```python
from build123d import *

# Parameters (mm, degrees)
F0_R     = 37
F0_R_2   = 3.25
F1_DEPTH = 4
F2_SIZE  = 2.75
F3_SIZE  = 0.5


with BuildPart() as f1:
    # F0 (on Top) → F1 (new body)
    with BuildSketch(Plane.XY):
        Circle(F0_R)
        with Locations((0, -29)):
            Circle(F0_R_2, mode=Mode.SUBTRACT)
        with Locations((-29, 0)):
            Circle(F0_R_2, mode=Mode.SUBTRACT)
        with Locations((29, 0)):
            Circle(F0_R_2, mode=Mode.SUBTRACT)
        with Locations((0, 29)):
            Circle(F0_R_2, mode=Mode.SUBTRACT)
    extrude(amount=F1_DEPTH)

    # F2
    f2_edges = [f1.edges().sort_by_distance(p)[0] for p in [
        (-3.25, -29, 4),
        (-32.25, 0, 4),
        (-3.25, 29, 4),
        (25.75, 0, 4),
    ]]
    chamfer(f2_edges, length=F2_SIZE)

    # F3
    f3_edges = [f1.edges().sort_by_distance(p)[0] for p in [
        (37, 0, 2),
        (-37, 0, 0),
        (-37, 0, 4),
        (-3.25, -29, 0),
        (-32.25, 0, 0),
        (-3.25, 29, 0),
        (25.75, 0, 0),
    ]]
    chamfer(f3_edges, length=F3_SIZE)


solid = f1.part
```
Verification items for the finished model (mm, model axes). Round coordinates to 2 decimals unless told otherwise and drop trailing zeros. Write each loop counter-clockwise with the first axis right and the second up, starting at its lowest first coordinate (ties: lowest second). Pieces come first, ordered by that corner, then holes. Notation, with made-up numbers: (-29.5, 34) - (-5.5, 34) arc R22 ccw to (-5.5, 48) - close; hole circle Ø9 at (20, 21.25). An arc over 180 degrees is marked (long way). Answer as a JSON object with one key per item and string values. Group by question number.
Q1. Section check C-C, the plane z = 2.45. Enter the section's corners in (x, y), plus the area to 3 significant figures.
Q2. Mould release check, pull along X, two halves, no side actions. Record for faces 1 (the cylindrical face through (-8.02, -36.12, 1.98)), 2 (the conical face through (32.26, 1.03, 1.42)), 3 (the flat face through (-1, 1, 0)): released by +X, released by -X, zero draft, split by the parting line, or undercut.
Q3. Section check A-A, the plane y = 0. Enter the section's corners in (x, z), plus the area to 3 significant figures.
Q4. Thickness scan on line 1 (Y direction, x = 0, z = 0.85); line 2 (X direction, y = 1, z = 1.7); line 3 (Y direction, x = 1.5, z = 3.6). Record the ranges inside material, lowest first.
Q5. Go/stop test with flat-tipped pins: pin 1 Ø1 at (x, y) = (-0.5, -5) entering from -Z; pin 2 Ø8.5 at (x, y) = (0, 29) entering from +Z; pin 3 Ø10.5 at (x, y) = (0, -29) entering from +Z; pin 4 Ø7.5 at (x, y) = (-29, 0) entering from +Z. Record where each tip stops, or that it passes through.
Found:
{
 "1": {"outline": "circle Ø74 at (0, 0); hole circle Ø8.9 at (-29, 0); hole circle Ø8.9 at (0, -29); hole circle Ø8.9 at (0, 29); hole circle Ø8.9 at (29, 0)", "area": "4,050 mm^2"},
 "2": {"face 1": "split by the parting line", "face 2": "undercut", "face 3": "zero draft"},
 "3": {"outline": "(-37, 0.5) - (-36.5, 0) - (-32.75, 0) - (-32.25, 0.5) - (-32.25, 1.25) - (-35, 4) - (-36.5, 4) - (-37, 3.5) - close; (-25.75, 0.5) - (-25.25, 0) - (25.25, 0) - (25.75, 0.5) - (25.75, 1.25) - (23, 4) - (-23, 4) - (-25.75, 1.25) - close; (32.25, 0.5) - (32.75, 0) - (36.5, 0) - (37, 0.5) - (37, 3.5) - (36.5, 4) - (35, 4) - (32.25, 1.25) - close", "area": "228 mm^2"},
 "4": {"line 1": "y = -37 to -32.25, -25.75 to 25.75, 32.25 to 37", "line 2": "x = -36.99 to -32.56, -25.44 to 25.44, 32.56 to 36.99", "line 3": "y = -36.87 to -34.4, -23.6 to 23.6, 34.4 to 36.87"},
 "5": {"pin 1": "stops at z = 0", "pin 2": "stops at z = 2.25", "pin 3": "stops at z = 3.25", "pin 4": "stops at z = 1.75"}
}
